```python
from build123d import *

# Parameters (mm, degrees)
SKETCH1_R           = 60
BOSS_EXTRUDE1_DEPTH = 10
SKETCH2_R           = 48.25
SKETCH2_R_2         = 38.25
BOSS_EXTRUDE2_DEPTH = 200
SKETCH3_R           = 43.25
CUT_EXTRUDE1_DEPTH  = 5


with BuildPart() as part:
    # Sketch1 → Boss-Extrude1 (new body)
    with BuildSketch(Plane(origin=(0, 0, 0), x_dir=(1, 0, 0), z_dir=(0, 1, 0))):
        with Locations(Location((0, 0, 0), (0, 0, 270))):
            Circle(SKETCH1_R)
    extrude(amount=BOSS_EXTRUDE1_DEPTH)

    # Sketch2 → Boss-Extrude2 (add)
    with BuildSketch(Plane(origin=(0, 10, 0), x_dir=(1, 0, 0), z_dir=(0, 1, 0))):
        with Locations(Location((0, 0, 0), (0, 0, 270))):
            Circle(SKETCH2_R)
        with Locations(Location((0, 0, 0), (0, 0, 270))):
            Circle(SKETCH2_R_2, mode=Mode.SUBTRACT)
    extrude(amount=BOSS_EXTRUDE2_DEPTH)

    # Sketch3 → Cut-Extrude1 (cut)
    with BuildSketch(Plane(origin=(0, 210, 0), x_dir=(1, 0, 0), z_dir=(0, 1, 0))):
        with Locations(Location((0, 0, 0), (0, 0, 270))):
            Circle(SKETCH3_R)
    extrude(amount=-CUT_EXTRUDE1_DEPTH, mode=Mode.SUBTRACT)


solid = part.part
```
Here's how the part is built. I have some questions about the finished solid (model axes, mm). A direction names the side the tool comes from. Give positions to 0.01 mm unless a question says otherwise; leave off trailing zeros. Loops run counter-clockwise (first coordinate to the right, second up) from the corner with the lowest first, then second, coordinate; pieces in that order, holes last. Notation, with made-up numbers: (16.25, 57) -> (60.25, 57) arc R17 ccw to (60.25, 62) -> close; hole circle Ø9 at (-36.5, -37.75). An arc over 180 degrees is marked (long way). Use one line per item in the form item = value. Start each with the question number.
1) For P1, Ø5, axis at x = -15, y = 45.5, coming from the +Z side; P2, Ø1.5, axis at x = 16.5, y = 183, coming from the +Z side; P3, Ø6, axis at x = -11.5, y = 158.5, coming from the +Z side, each with a flat end and sliding along its axis, tell me the tip position at first contact or that it passes through.
2) Please list where these lines run through material, in increasing order: line 1 along X through (y, z) = (80, 0); line 2 along X through (y, z) = (206.8, 0); line 3 along Y through (x, z) = (19, -38).
3) Imagine slicing it at C-C (z = 0). Please give me the cut outline in (x, y).
4) Imagine slicing it at A-A (x = 0). Please give me the cut outline in (y, z), then the cut area to 3 significant figures.
5) Which directions (+Z, -Z, +X, -X, +Y, -Y) give clear straight access to the entire face, cutting with the end or side of a thin tool? Please do faces 1 (the face through (2.64, 4.93, -59.94)), 2 (the face through (1, 10, -1)).
6) Thinking about a two-plate mould opening in Z: for faces 3 (the face through (-37.34, 106.14, -8.29)), 4 (the face through (-35, 205, 16)), 5 (the face through (-47.103, 108.6, -10.46)), 6 (the face through (1, 0, -1)), which applies, +Z half, -Z half, draft (parallel to the pull), parting line (faces both ways), or undercut?
7) Imagine slicing it at B-B (y = 151.5). Please give me the cut outline in (x, z), then the cut area to 3 significant figures.
Check values:
q1.P1 = 46.6
q1.P2 = 45.61
q1.P3 = 47.5
q2.line_1 = -48.25 to -38.25, 38.25 to 48.25
q2.line_2 = -48.25 to -43.25, 43.25 to 48.25
q2.line_3 = 0 to 205
q3.outline = (-60, 0) -> (60, 0) -> (60, 10) -> (48.25, 10) -> (48.25, 210) -> (43.25, 210) -> (43.25, 205) -> (38.25, 205) -> (38.25, 10) -> (-38.25, 10) -> (-38.25, 205) -> (-43.25, 205) -> (-43.25, 210) -> (-48.25, 210) -> (-48.25, 10) -> (-60, 10) -> close
q4.outline = (0, -60) -> (10, -60) -> (10, -48.25) -> (210, -48.25) -> (210, -43.25) -> (205, -43.25) -> (205, -38.25) -> (10, -38.25) -> (10, 38.25) -> (205, 38.25) -> (205, 43.25) -> (210, 43.25) -> (210, 48.25) -> (10, 48.25) -> (10, 60) -> (0, 60) -> close
q4.area = 5,150 mm^2
q5.face_1 = +Y, -Y
q5.face_2 = +Y
q6.face_3 = undercut
q6.face_4 = undercut
q6.face_5 = parting line
q6.face_6 = draft
q7.outline = circle Ø96.5 at (0, 0); hole circle Ø76.5 at (0, 0)
q7.area = 2,720 mm^2
